For this review, use the dimensioned drawing (mm, ordinates from the lowest corner) and the shaded views. Coordinates: 2 decimals unless noted, no trailing zeros. Write each loop counter-clockwise with the first axis right and the second up, starting at its lowest first coordinate (ties: lowest second). Pieces come first, ordered by that corner, then holes. Notation, with made-up numbers: (-33, -32.5) - (6, -32.5) arc R16 ccw to (6, -16.5) - close; hole circle Ø2 at (43, 73). An arc over 180 degrees is marked (long way). Put each result on its own line as item: value.
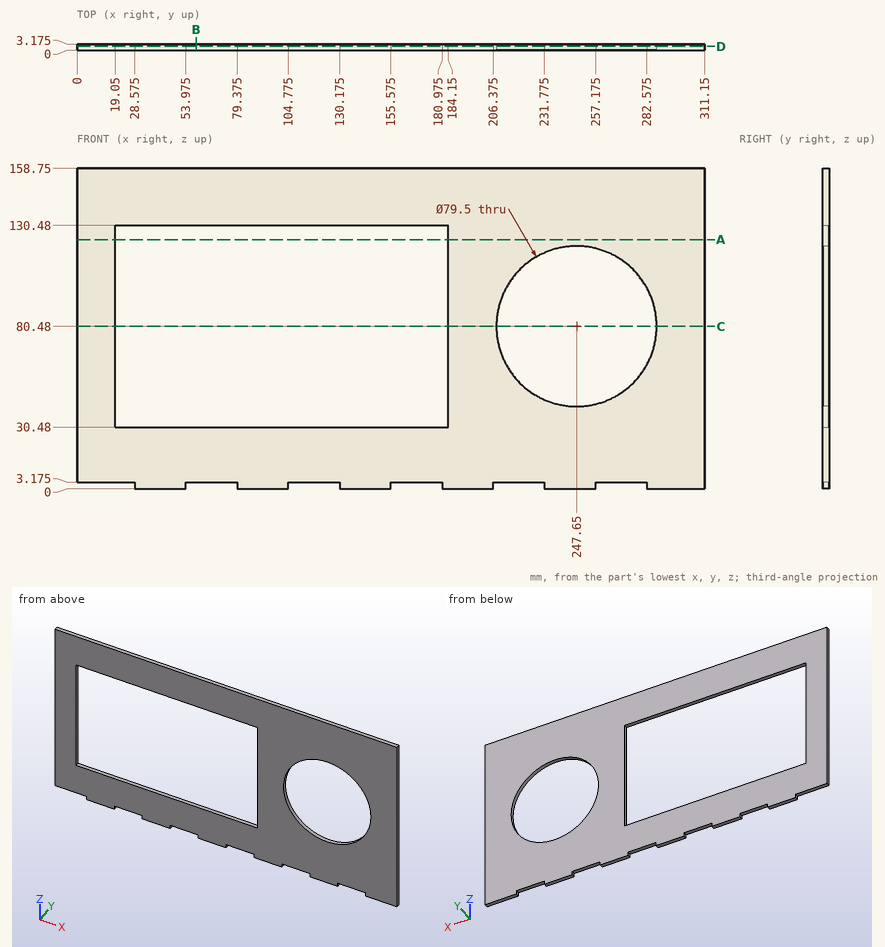
1. Consider section C-C on z = 80.48. State the section outline as (x, y) points (3 decimals).
Determined:
outline: (0, 0) - (19.05, 0) - (19.05, 3.175) - (0, 3.175) - close; (184.15, 0) - (207.9, 0) - (207.9, 3.175) - (184.15, 3.175) - close; (287.4, 0) - (311.15, 0) - (311.15, 3.175) - (287.4, 3.175) - close
2. Consider section A-A on z = 123.5. State the section outline as (x, y) points (3 decimals), plus the area to 3 significant figures.
Determined:
outline: (0, 0) - (19.05, 0) - (19.05, 3.175) - (0, 3.175) - close; (184.15, 0) - (311.15, 0) - (311.15, 3.175) - (184.15, 3.175) - close
area: 464 mm^2
3. To check wall thickness, follow probe 1 along X at (y, z) = (2, 59.5); probe 2 along Z at (x, y) = (62, 3.05) (3 decimals); probe 3 along X at (y, z) = (1.25, 60.5). State the ranges of each line that lie inside material, in increasing order.
Determined:
probe 1: x = 0 to 19.05, 184.15 to 213.89, 281.41 to 311.15
probe 2: z = 3.175 to 30.48, 130.48 to 158.75
probe 3: x = 0 to 19.05, 184.15 to 213.29, 282.01 to 311.15
4. Consider section D-D on y = 2. Give the number of separate pieces and of enclosed holes in the cut face, plus the area to 3 significant figures.
Determined:
separate pieces: 1
enclosed holes: 2
area: 27,400 mm^2
5. For pin 1 Ø1.6 at (y, z) = (1, 2) entering from -X (3 decimals); pin 2 Ø1 at (x, z) = (279.5, 59) entering from +Y; pin 3 Ø1.6 at (x, y) = (123.5, 2) entering from -Z (3 decimals), all flat-tipped, find the tip position at first contact; note any pin that passes through.
Determined:
pin 1: stops at x = 28.575
pin 2: passes through
pin 3: stops at z = 3.175
6. Consider section B-B on x = 59. State the section outline as (y, z) points (3 decimals), plus the area to 3 significant figures.
Determined:
outline: (0, 3.175) - (3.175, 3.175) - (3.175, 30.48) - (0, 30.48) - close; (0, 130.48) - (3.175, 130.48) - (3.175, 158.75) - (0, 158.75) - close
area: 176 mm^2
